Part model, mm, in its own coordinate system. Round coordinates to 2 decimals unless told otherwise and drop trailing zeros. Order: outer loops, then holes, each group sorted by start corner. A loop starts at its lowest first (then second) coordinate and runs counter-clockwise, first axis right, second up. Notation, with made-up numbers: M 61.5,82 L 67.5,82 A22 ccw 67.5,97 Z; hole C 1,44 d9. An arc over 180 degrees is marked long. One line per question, with ' | ' between items.
from build123d import *


with BuildPart() as cone:
    # Cone → Cone (revolve)
    with BuildSketch(Plane.XZ):
        Polygon((0, 0), (4, 0), (0, 10), align=None)
    revolve(axis=Axis((0, 0, 0), (0, 0, 1)))


with BuildPart() as fusion:
    # Sphere001 → Sphere001 (revolve)
    with BuildSketch(Plane.XZ):
        with BuildLine():
            ThreePointArc((0, -5), (5, 0), (0, 5))
            Line((0, 5), (0, -5))
        make_face()
    revolve(axis=Axis((0, 0, 0), (0, 0, 1)))

    # Fusion: union Cone
    add(cone.part)


solid = fusion.part
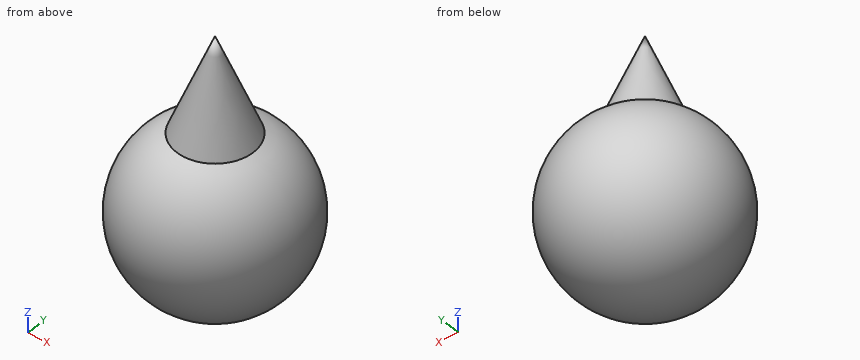
1) Probe line 1 (Y direction, x = 2, z = -1); line 2 (Y direction, x = 3, z = -1.5); line 3 (Z direction, x = -0.5, y = 3.5). List the from-to ranges inside material, lowest first. Write a range as [from, to].
The answers:
line 1: y = [-4.47, 4.47] | line 2: y = [-3.71, 3.71] | line 3: z = [-3.54, 3.54]
2) Saw through at A-A (z = 9.25). List the corners of the cut face in (x, y).
The answers:
outline: C 0,0 d0.6
3) Drop flat-ended pins along their axis: pin 1 (1.5 mm diameter, centred on x = -3, y = 2, fed in from +Z); pin 2 (6 mm diameter, centred on x = 2, y = 2, fed in from +Z); pin 3 (1.5 mm diameter, centred on y = -3.5, z = 0, fed in from +X); pin 4 (1.5 mm diameter, centred on x = -0.5, z = 6, fed in from -Y). Give the stop position or say it passes through.
The answers:
pin 1: stops at z = 4.1 | pin 2: stops at z = 10 | pin 3: stops at x = 4.18 | pin 4: stops at y = -1.87
4) Saw through at B-B (y = 4). List the corners of the cut face in (x, z).
The answers:
outline: C 0,0 d6
